```python
from build123d import *

# Parameters (mm, degrees)
SKETCH1_W                      = 220
SKETCH1_H                      = 158
BOSS_EXTRUDE1_DEPTH            = 5.5
CBORE_FOR_M4_SHCS1_D           = 4.5
CBORE_FOR_M4_SHCS1_CBORE_D     = 8
CBORE_FOR_M4_SHCS1_CBORE_DEPTH = 4
SKETCH6_W                      = 20
SKETCH6_H                      = 40
CUT_EXTRUDE2_DEPTH             = 6.5


with BuildPart() as part:
    # Sketch1 → Boss-Extrude1 (new body)
    with BuildSketch(Plane(origin=(0, 0, 0), x_dir=(1, 0, 0), z_dir=(0, 1, 0))):
        Rectangle(SKETCH1_W, SKETCH1_H)
    extrude(amount=BOSS_EXTRUDE1_DEPTH)

    # CBORE for M4 SHCS1 (through all)
    with Locations(Plane.XZ):
        with Locations((100, 0)):
            cbore_for_m4_shcs1 = CounterBoreHole(CBORE_FOR_M4_SHCS1_D / 2, CBORE_FOR_M4_SHCS1_CBORE_D / 2, CBORE_FOR_M4_SHCS1_CBORE_DEPTH)

    # Mirror2: CBORE for M4 SHCS1 across plane
    add(cbore_for_m4_shcs1.mirror(Plane(origin=(0, 0, 0), x_dir=(0, 0, 1), z_dir=(1, 0, 0))), mode=Mode.SUBTRACT)

    # Sketch6 → Cut-Extrude2 (cut, through all)
    with BuildSketch(Plane(origin=(0, 5.5, 0), x_dir=(1, 0, 0), z_dir=(0, 1, 0))):
        with Locations((100, 59)):
            Rectangle(SKETCH6_W, SKETCH6_H)
    extrude(amount=-CUT_EXTRUDE2_DEPTH, mode=Mode.SUBTRACT)


solid = part.part
```
Geometry check sheet. Reference: the model listing, model coordinates, mm. A direction names the side the tool comes from. Give positions to 0.01 mm unless a question says otherwise; leave off trailing zeros. Loops run counter-clockwise (first coordinate to the right, second up) from the corner with the lowest first, then second, coordinate; pieces in that order, holes last. Notation, with made-up numbers: (-13.75, -8.5) - (34.25, -8.5) arc R25 cw to (34.25, 24.5) - close; hole circle Ø5 at (29.25, 84.25). An arc over 180 degrees is marked (long way). Use CSV: the item, a comma, the result in double quotes. Start each with the question number.
Q1. Go/stop test with a flat-tipped pin: pin 1 Ø5 at (x, z) = (-100, 0) entering from -Y. Record where the tip stops, or that it passes through.
Q2. Section check C-C, the plane y = 2.95. Record the cut outline in (x, z).
Q3. Section check B-B, the plane z = 0. Record the cut outline in (x, y), and give its area (3 significant figures).
Q4. Section check A-A, the plane x = 100. Record the cut outline in (y, z), and give its area (3 significant figures).
Q5. Scan lines: probe 1 along Z at (x, y) = (100, 4.6); probe 2 along Z at (x, y) = (-100, 4.8); probe 3 along Z at (x, y) = (95, 2.8). Record each from-to range of solid material in increasing order. Write a range as from..to.
Q6. Release check for a two-part mould opening along Z. For faces 1 (the face through (102, 4, -2)), 2 (the face through (-11, 3, -79)), 3 (the face through (90, 3, -59)), 4 (the face through (-2, 3, 79)) record: +Z half, -Z half, draft (parallel to the pull), parting line (faces both ways), or undercut.
Q7. Section check D-D, the plane x = -100. Record the cut outline in (y, z).
Q8. Access from +Z, -Z, +X, -X, +Y, -Y to the whole of each face (thin tool, end or side, straight path). Record for faces 5 (the face through (103.695, 1.972, -1.532)), 6 (the face through (100, 3, -39)), 7 (the face through (-2, 5.5, -1)).
Findings below:
1,pin 1,"stops at y = 4"
2,outline,"(-110, -79) - (90, -79) - (90, -39) - (110, -39) - (110, 79) - (-110, 79) - close; hole circle Ø8 at (-100, 0); hole circle Ø8 at (100, 0)"
3,outline,"(-110, 0) - (-104, 0) - (-104, 4) - (-102.25, 4) - (-102.25, 5.5) - (-110, 5.5) - close; (-97.75, 4) - (-96, 4) - (-96, 0) - (96, 0) - (96, 4) - (97.75, 4) - (97.75, 5.5) - (-97.75, 5.5) - close; (102.25, 4) - (104, 4) - (104, 0) - (110, 0) - (110, 5.5) - (102.25, 5.5) - close"
3,area,"1,130 mm^2"
4,outline,"(0, -39) - (5.5, -39) - (5.5, -2.25) - (4, -2.25) - (4, -4) - (0, -4) - close; (0, 4) - (4, 4) - (4, 2.25) - (5.5, 2.25) - (5.5, 79) - (0, 79) - close"
4,area,"610 mm^2"
5,probe 1,"z = -39..-2.25, 2.25..79"
5,probe 2,"z = -79..-2.25, 2.25..79"
5,probe 3,"z = -39..79"
6,face 1,"undercut"
6,face 2,"-Z half"
6,face 3,"draft"
6,face 4,"+Z half"
7,outline,"(0, -79) - (5.5, -79) - (5.5, -2.25) - (4, -2.25) - (4, -4) - (0, -4) - close; (0, 4) - (4, 4) - (4, 2.25) - (5.5, 2.25) - (5.5, 79) - (0, 79) - close"
8,face 5,"-Y"
8,face 6,"-Z, +X, +Y, -Y"
8,face 7,"+Z, -Z, +X, -X, +Y"
